Check sheet for the modelled part. Datum: model origin and axes. Units: mm. A direction names the side the tool comes from. Coordinates: 2 decimals unless noted, no trailing zeros. Order: outer loops, then holes, each group sorted by start corner. A loop starts at its lowest first (then second) coordinate and runs counter-clockwise, first axis right, second up.
from build123d import *

# Parameters (mm, degrees)
SKETCH1_R           = 114.3
BOSS_EXTRUDE1_DEPTH = 6.35
SKETCH2_W           = 6.35
SKETCH2_H           = 114.3
CUT_EXTRUDE1_DEPTH  = 6.35
CUT_EXTRUDE2_DEPTH  = 162.769287876
SKETCH4_R           = 3.175
CUT_EXTRUDE3_DEPTH  = 162.769287876


with BuildPart() as part:
    # Sketch1 → Boss-Extrude1 (new body)
    with BuildSketch(Plane(origin=(0, 0, 0), x_dir=(1, 0, 0), z_dir=(0, 1, 0))):
        with Locations(Location((0, 0, 0), (0, 0, 270))):
            Circle(SKETCH1_R)
    extrude(amount=BOSS_EXTRUDE1_DEPTH)

    # Sketch2 → Cut-Extrude1 (cut)
    with BuildSketch(Plane(origin=(0, 6.35, 0), x_dir=(1, 0, 0), z_dir=(0, 1, 0))):
        with Locations((0, -57.15)):
            Rectangle(SKETCH2_W, SKETCH2_H)
    extrude(amount=-CUT_EXTRUDE1_DEPTH, mode=Mode.SUBTRACT)

    # Sketch3 → Cut-Extrude2 (cut, through all)
    with BuildSketch(Plane(origin=(0, 6.35, 0), x_dir=(1, 0, 0), z_dir=(0, 1, 0))):
        Polygon((114.255894268, 3.175), (120.605894268, 3.175), (120.605894268, -3.175), (114.255894268, -3.175), (50.755894268, -3.175), (50.755894268, 3.175), align=None)
    extrude(amount=-CUT_EXTRUDE2_DEPTH, mode=Mode.SUBTRACT)

    # Sketch4 → Cut-Extrude3 (cut, through all)
    with BuildSketch(Plane(origin=(0, 6.35, 0), x_dir=(1, 0, 0), z_dir=(0, 1, 0))):
        with Locations(Location((101.6, -12.7, 0), (0, 0, 270))):
            Circle(SKETCH4_R)
        with Locations(Location((-101.6, -12.7, 0), (0, 0, 270))):
            Circle(SKETCH4_R)
    extrude(amount=-CUT_EXTRUDE3_DEPTH, mode=Mode.SUBTRACT)


solid = part.part
(1) Go/stop test with flat-tipped pins: P1, Ø1.9, axis at x = 89, y = 2, coming from the -Z side; P2, Ø2, axis at y = 2.5, z = -85.5, coming from the -X side; P3, Ø1.9, axis at x = -0.5, y = 3.5, coming from the +Z side. Record where each tip stops, or that it passes through.
Filled in:
P1: stops at z = -72.88
P2: stops at x = -76.97
P3: stops at z = 0
(2) Cross-section at B-B (z = 62). Enter the section's corners in (x, y) (3 decimals), and give its area (3 significant figures).
Filled in:
outline: (-96.023, 0) - (-3.175, 0) - (-3.175, 6.35) - (-96.023, 6.35) - close; (3.175, 0) - (96.023, 0) - (96.023, 6.35) - (3.175, 6.35) - close
area: 1,180 mm2
(3) Thickness scan on probe 1 along X at (y, z) = (4, 12.7) (3 decimals); probe 2 along X at (y, z) = (4.5, 14) (3 decimals); probe 3 along X at (y, z) = (4.25, 2) (1 decimal). Record the ranges inside material, lowest first.
Filled in:
probe 1: x = -113.592 to -104.775, -98.425 to -3.175, 3.175 to 98.425, 104.775 to 113.592
probe 2: x = -113.439 to -104.497, -98.703 to -3.175, 3.175 to 98.703, 104.497 to 113.439
probe 3: x = -114.3 to -3.2, 3.2 to 50.8
(4) Tool access check on faces 5 (the flat face through (82, 3, 3.175)), 6 (the flat face through (0, 3, 0)), 7 (the cylindrical face through (-78.15, 3.13, -83.41)). Record the directions out of +Z, -Z, +X, -X, +Y, -Y that give a thin tool (end or side, any length) a straight path to the whole face; none if there is none.
Filled in:
face 5: +X, +Y, -Y
face 6: +Z, +Y, -Y
face 7: +Y, -Y
(5) Release check for a two-part mould opening along X. For faces 1 (the cylindrical face through (79.961, 3.131, 81.675)), 2 (the flat face through (2, 6.35, -2)), 3 (the flat face through (-3.175, 3, 58)), 4 (the flat face through (3.175, 3, 58)) record: +X half, -X half, draft (parallel to the pull), parting line (faces both ways), or undercut.
Filled in:
face 1: +X half
face 2: draft
face 3: undercut
face 4: undercut
(6) Cross-section at C-C (y = 4.25). Enter the section's corners in (x, z) (3 decimals), and give its area (3 significant figures).
Filled in:
outline: (-3.175, 0) - (-3.175, 114.256) arc R114.3 ccw (long way) to (114.256, -3.175) - (50.756, -3.175) - (50.756, 3.175) - (114.256, 3.175) arc R114.3 ccw to (3.175, 114.256) - (3.175, 0) - close; hole circle Ø6.35 at (-101.6, 12.7); hole circle Ø6.35 at (101.6, 12.7)
area: 39,900 mm2
(7) Cross-section at D-D (z = 12.7). Enter the section's corners in (x, y) (3 decimals).
Filled in:
outline: (-113.592, 0) - (-104.775, 0) - (-104.775, 6.35) - (-113.592, 6.35) - close; (-98.425, 0) - (-3.175, 0) - (-3.175, 6.35) - (-98.425, 6.35) - close; (3.175, 0) - (98.425, 0) - (98.425, 6.35) - (3.175, 6.35) - close; (104.775, 0) - (113.592, 0) - (113.592, 6.35) - (104.775, 6.35) - close
(8) Cross-section at A-A (x = -101.6). Enter the section's corners in (y, z) (3 decimals), and give its area (3 significant figures).
Filled in:
outline: (0, -52.363) - (6.35, -52.363) - (6.35, 9.525) - (0, 9.525) - close; (0, 15.875) - (6.35, 15.875) - (6.35, 52.363) - (0, 52.363) - close
area: 625 mm2
